The model under review builds one solid part; all positions refer to its coordinate system, in mm. Face numbers are marked on the shaded views. Coordinates: 2 decimals unless noted, no trailing zeros. Order: outer loops, then holes, each group sorted by start corner. A loop starts at its lowest first (then second) coordinate and runs counter-clockwise, first axis right, second up. Notation, with made-up numbers: (36, -39) -> (59, -39) arc R5 ccw to (59, -35) -> close; hole circle Ø1 at (76.25, 33.25). An arc over 180 degrees is marked (long way). Use one line per item in the form item = value. Start each with the question number.
(1) Take a section at B-B (z = 2.6). State how many separate pieces and enclosed holes the cut face has, then the cut area to 3 significant figures.
(2) Insertion check: pin 1 Ø1.5 at (x, z) = (43, 1.5) entering from +Y. The pin has a flat end and moves straight along its axis. Give the tip position at first contact, or say it passes through.
(3) Take a section at C-C (x = 11). State the section outline as (y, z) points (3 decimals), then the cut area to 3 significant figures.
(4) Take a section at A-A (y = 19.05). State the section outline as (x, z) points (1 decimal).
(5) Wall thickness on line 1 along X through (y, z) = (17.25, 0.2); line 2 along Y through (x, z) = (37, 1.75); line 3 along X through (y, z) = (13, 1): over which ranges is each line inside the solid? List them lowest first.
(6) Mouldability with a two-part tool opening along X and no side actions: class the marked faces 1, 2 and 3 as +X half, -X half, draft (parallel to the pull), parting line (faces both ways), or undercut.
(7) Take a section at D-D (y = 23). State the section outline as (x, z) points (3 decimals), then the cut area to 3 significant figures.
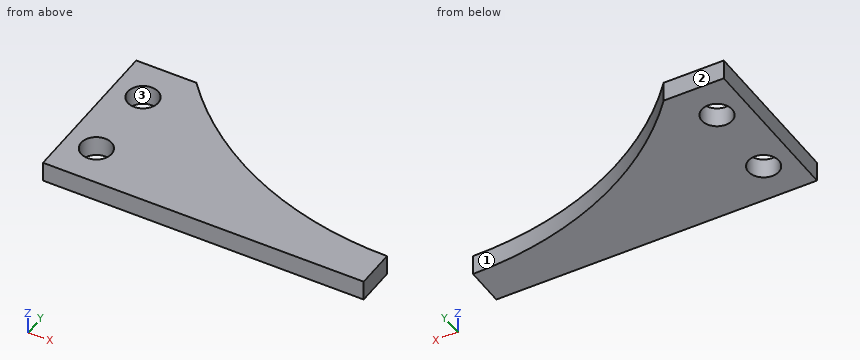
```python
from build123d import *

# Parameters (mm, degrees)
SKETCH1_R           = 2.413
BOSS_EXTRUDE1_DEPTH = 3.175


with BuildPart() as part:
    # Sketch1 → Boss-Extrude1 (new body)
    with BuildSketch(Plane.XY):
        with BuildLine():
            Line((0, 0), (0, 25.4))
            Line((0, 25.4), (9.525, 25.4))
            ThreePointArc((9.525, 25.4), (28.070459062, 11.342244634), (50.8, 6.35))
            Line((50.8, 6.35), (50.8, 0))
            Line((50.8, 0), (0, 0))
        make_face()
        with Locations((4.7625, 6.35)):
            Circle(SKETCH1_R, mode=Mode.SUBTRACT)
        with Locations((4.7625, 19.05)):
            Circle(SKETCH1_R, mode=Mode.SUBTRACT)
    extrude(amount=BOSS_EXTRUDE1_DEPTH)


solid = part.part
```
Findings:
q1.separate_pieces = 1
q1.enclosed_holes = 2
q1.area = 708 mm²
q2.pin_1 = 7.03
q3.outline = (0, 0) -> (23.74, 0) -> (23.74, 3.175) -> (0, 3.175) -> close
q3.area = 75.4 mm²
q4.outline = (0, 0) -> (2.3, 0) -> (2.3, 3.2) -> (0, 3.2) -> close; (7.2, 0) -> (15.9, 0) -> (15.9, 3.2) -> (7.2, 3.2) -> close
q5.line_1 = 0 to 3.16, 6.37 to 18.19
q5.line_2 = 0 to 8.13
q5.line_3 = 0 to 24.78
q6.face_1 = +X half
q6.face_2 = draft
q6.face_3 = undercut
q7.outline = (0, 0) -> (11.698, 0) -> (11.698, 3.175) -> (0, 3.175) -> close
q7.area = 37.1 mm²
